from build123d import *

# Parameters (mm, degrees)
EXTRUDE_1_DEPTH      = 1.25
EXTRUDE_1_DEPTH_BACK = 1.25
SKETCH_1_R           = 2
SKETCH_1_R_2         = 1.5
EXTRUDE_2_DEPTH      = 1
EXTRUDE_2_DEPTH_BACK = 1
SKETCH_2_R           = 2.5
SKETCH_2_R_2         = 2
EXTRUDE_3_DEPTH      = 1.25
EXTRUDE_3_DEPTH_BACK = 1.25
SKETCH_3_R           = 3
SKETCH_3_R_2         = 2.5


with BuildPart() as part:
    # Sketch 1 → Extrude 1 (new, two sides: drawn at the far end of the back side and taken through both)
    with BuildSketch(Plane(origin=(0, 0, 0), x_dir=(1, 0, 0), z_dir=(0, 1, 0)).offset(-EXTRUDE_1_DEPTH_BACK)):
        with Locations(Location((0, 0, 0), (0, 0, 270))):
            Circle(SKETCH_1_R)
        with Locations(Location((0, 0, 0), (0, 0, 270))):
            Circle(SKETCH_1_R_2, mode=Mode.SUBTRACT)
    extrude(amount=EXTRUDE_1_DEPTH + EXTRUDE_1_DEPTH_BACK)

    # Sketch 2 → Extrude 2 (add, two sides: drawn at the far end of the back side and taken through both)
    with BuildSketch(Plane(origin=(0, 0, 0), x_dir=(1, 0, 0), z_dir=(0, 1, 0)).offset(-EXTRUDE_2_DEPTH_BACK)):
        with Locations(Location((0, 0, 0), (0, 0, 270))):
            Circle(SKETCH_2_R)
        with Locations(Location((0, 0, 0), (0, 0, 270))):
            Circle(SKETCH_2_R_2, mode=Mode.SUBTRACT)
    extrude(amount=EXTRUDE_2_DEPTH + EXTRUDE_2_DEPTH_BACK)

    # Sketch 3 → Extrude 3 (add, two sides: drawn at the far end of the back side and taken through both)
    with BuildSketch(Plane(origin=(0, 0, 0), x_dir=(1, 0, 0), z_dir=(0, 1, 0)).offset(-EXTRUDE_3_DEPTH_BACK)):
        with Locations(Location((0, 0, 0), (0, 0, 270))):
            Circle(SKETCH_3_R)
        with Locations(Location((0, 0, 0), (0, 0, 270))):
            Circle(SKETCH_3_R_2, mode=Mode.SUBTRACT)
    extrude(amount=EXTRUDE_3_DEPTH + EXTRUDE_3_DEPTH_BACK)


solid = part.part
Geometry check sheet. Reference: the model listing, model coordinates, mm. A direction names the side the tool comes from. Round coordinates to 2 decimals unless told otherwise and drop trailing zeros. Order: outer loops, then holes, each group sorted by start corner. A loop starts at its lowest first (then second) coordinate and runs counter-clockwise, first axis right, second up. Notation, with made-up numbers: M -4,64 L 37,64 A20 ccw 37,97 Z; hole C -28.75,-20 d2. An arc over 180 degrees is marked long. Answer in a Markdown table with one row per item. Add a question column.
Item 1: Material ranges on L1, parallel to X at y = -1.2, z = 0; L2, parallel to X at y = -0.1, z = 0; L3, parallel to Z at x = -0.6, y = -1.05, recorded low to high. Write a range as [from, to].
Item 2: Sectioned sample at A-A, the plane x = 0. Enter the section's corners in (y, z).
Item 3: Set-up check for faces 4 (the face through (2, 1.25, -2)), 5 (the face through (2, 1, -1)): record each of +Z, -Z, +X, -X, +Y, -Y from which the full face is reachable in a straight line by a thin tool's end or side.
Item 4: Draft check along X on faces 1 (the face through (0.9, -0.02, 2.86)), 2 (the face through (2, -1.25, -2)), 3 (the face through (2, -1, -1)). Enter one of: released by +X, released by -X, zero draft, split by the parting line, or undercut.
Item 5: Sectioned sample at B-B, the plane z = 0. Enter the section's corners in (x, y).
Item 6: Sectioned sample at D-D, the plane y = -0.9. Enter the section's corners in (x, z).
Item 7: Sectioned sample at C-C, the plane y = 1.1. Enter the section's corners in (x, z), plus the area to 3 significant figures.
Filled in:
| question | item | result |
|---|---|---|
| 1 | L1 | x = [-3, -2.5], [-2, -1.5], [1.5, 2], [2.5, 3] |
| 1 | L2 | x = [-3, -1.5], [1.5, 3] |
| 1 | L3 | z = [-2.94, -2.43], [-1.91, -1.37], [1.37, 1.91], [2.43, 2.94] |
| 2 | outline | M -1.25,-3 L 1.25,-3 L 1.25,-2.5 L 1,-2.5 L 1,-2 L 1.25,-2 L 1.25,-1.5 L -1.25,-1.5 L -1.25,-2 L -1,-2 L -1,-2.5 L -1.25,-2.5 Z; M -1.25,1.5 L 1.25,1.5 L 1.25,2 L 1,2 L 1,2.5 L 1.25,2.5 L 1.25,3 L -1.25,3 L -1.25,2.5 L -1,2.5 L -1,2 L -1.25,2 Z |
| 3 | face 4 | +Z, -Z, +X, -X, +Y |
| 3 | face 5 | +Y |
| 4 | face 1 | split by the parting line |
| 4 | face 2 | zero draft |
| 4 | face 3 | undercut |
| 5 | outline | M -3,-1.25 L -2.5,-1.25 L -2.5,-1 L -2,-1 L -2,-1.25 L -1.5,-1.25 L -1.5,1.25 L -2,1.25 L -2,1 L -2.5,1 L -2.5,1.25 L -3,1.25 Z; M 1.5,-1.25 L 2,-1.25 L 2,-1 L 2.5,-1 L 2.5,-1.25 L 3,-1.25 L 3,1.25 L 2.5,1.25 L 2.5,1 L 2,1 L 2,1.25 L 1.5,1.25 Z |
| 6 | outline | C 0,0 d6; hole C 0,0 d3 |
| 7 | outline | C 0,0 d6; C 0,0 d4; hole C 0,0 d5; hole C 0,0 d3 |
| 7 | area | 14.1 mm² |
